from build123d import *

# Parameters (mm, degrees)
F0_R           = 8
F1_DEPTH       = 10
F2_SIZE        = 4
F3_SIZE        = 4
F4_D           = 3.3
F4_CSINK_D     = 6.72
F4_CSINK_ANGLE = 90
F6_D           = 5
F6_DEPTH       = 8
F6_TIP         = 1.5021515476


with BuildPart() as f1:
    # F0 (on Front) → F1 (new body)
    with BuildSketch(Plane.XZ):
        Polygon((-10, 0), (0, 0), (10, 0), (10, -10), (30, -10), (30, 0), (50, 0), (50, -10), (70, -10), (70, 0), (90, 0), (90, 15), (70, 15), (21, 258), (21, 300), (0, 300), (-21, 300), (-21, 258), (-70, 15), (-90, 15), (-90, 0), (-70, 0), (-70, -10), (-50, -10), (-50, 0), (-30, 0), (-30, -10), (-10, -10), align=None)
        with BuildLine():
            ThreePointArc((7.5, 50), (0, 42.5), (-7.5, 50))
            Line((-7.5, 50), (-7.5, 199.0483840028))
            ThreePointArc((-7.5, 199.0483840028), (0, 207.5601304887), (7.5, 199.0483840028))
            Line((7.5, 199.0483840028), (7.5, 50))
        make_face(mode=Mode.SUBTRACT)
        with Locations((0, 279)):
            Circle(F0_R, mode=Mode.SUBTRACT)
    extrude(amount=F1_DEPTH)

    # F2
    f2_edges = [f1.edges().sort_by_distance(p)[0] for p in [
        (21, -5, 300),
        (-21, -5, 300),
    ]]
    chamfer(f2_edges, length=F2_SIZE)

    # F3
    f3_edges = [f1.edges().sort_by_distance(p)[0] for p in [
        (-90, -5, 15),
        (90, -5, 15),
    ]]
    chamfer(f3_edges, length=F3_SIZE)

    # F4 (through all)
    with Locations(Plane(origin=(0, 0, 0), x_dir=(1, 0, 0), z_dir=(0, 1, 0))):
        with Locations((-15.5, -294.5), (15.5, -294.5), (15.5, -263.5), (-15.5, -263.5)):
            CounterSinkHole(F4_D / 2, F4_CSINK_D / 2, counter_sink_angle=F4_CSINK_ANGLE)

    # F6
    with Locations(Plane(origin=(0, 0, 0), x_dir=(1, 0, 0), z_dir=(0, 0, -1))):
        with Locations((-80, 5), (80, 5)):
            Hole(F6_D / 2, depth=F6_DEPTH)
            with Locations((0, 0, -(F6_DEPTH + F6_TIP / 2))):  # 118° drill point
                Cone(0, F6_D / 2, F6_TIP, mode=Mode.SUBTRACT)


solid = f1.part
Build history of the part. All positions in model axes, mm. A direction names the side the tool comes from. Round coordinates to 2 decimals unless told otherwise and drop trailing zeros. Write each loop counter-clockwise with the first axis right and the second up, starting at its lowest first coordinate (ties: lowest second). Pieces come first, ordered by that corner, then holes. Notation, with made-up numbers: (-26, 76.25) -> (-8, 76.25) arc R13 cw to (-8, 80.25) -> close; hole circle Ø2 at (8, -30). An arc over 180 degrees is marked (long way). Use one line per item in the form item = value.
Q1. Drill centre lines: L1, parallel to Z at x = 15.5, y = -6; L2, parallel to Y at x = 80, z = 6; L3, parallel to Z at x = -83, y = -9. Where is each one in solid material? Low to high.
Conclusion:
L1 = -10 to 261.85, 265.15 to 292.85, 296.15 to 300
L2 = -10 to -7.5, -2.5 to 0
L3 = 0 to 15
Q2. Band-saw the part on C-C, the plane x = -35. Write the cut outline in (y, z), then the cut area to 3 significant figures.
Conclusion:
outline = (-10, 0) -> (0, 0) -> (0, 188.57) -> (-10, 188.57) -> close
area = 1,890 mm²
Q3. Tool access for faces 1 (the flat face through (-78, -5, 15)), 2 (the cylindrical face through (0.16, -4.93, 42.5)), 3 (the flat face through (-30, -5, -5)): list every direction of +Z, -Z, +X, -X, +Y, -Y with a clear straight run to the whole face (end or side of a thin tool).
Conclusion:
face_1 = +Z, -X, +Y, -Y
face_2 = +Y, -Y
face_3 = -Z, +Y, -Y
Q4. Drop flat-ended pins along their axis: P1, Ø5, axis at y = -7, z = 272.5, coming from the +X side; P2, Ø4, axis at y = -6.5, z = 201, coming from the +X side; P3, Ø3, axis at x = -36.5, y = -7, coming from the -Z side; P4, Ø2, axis at x = 15.5, z = 294.5, coming from the -Y side. Give the stop position or say it passes through.
Conclusion:
P1 = 21
P2 = 32.9
P3 = 0
P4 = through
Q5. Band-saw the part on D-D, the plane z = 37. Write the cut outline in (x, y).
Conclusion:
outline = (-65.56, -10) -> (65.56, -10) -> (65.56, 0) -> (-65.56, 0) -> close
Q6. Two-plate mould, pull along X, no slides. Class faces 4 (the flat face through (-90, -5, 6)), 5 (the flat face through (40, -5, 0)), 6 (the flat face through (21, -5, 277)): released by +X, released by -X, zero draft, split by the parting line, or undercut.
Conclusion:
face_4 = released by -X
face_5 = undercut
face_6 = released by +X
Q7. Band-saw the part on A-A, the plane z = 279. Write the cut outline in (x, y), then the cut area to 3 significant figures.
Conclusion:
outline = (-21, -10) -> (-8, -10) -> (-8, 0) -> (-21, 0) -> close; (8, -10) -> (21, -10) -> (21, 0) -> (8, 0) -> close
area = 260 mm²
Q8. Band-saw the part on B-B, the plane z = 122. Write the cut outline in (x, y), then the cut area to 3 significant figures.
Conclusion:
outline = (-48.42, -10) -> (-7.5, -10) -> (-7.5, 0) -> (-48.42, 0) -> close; (7.5, -10) -> (48.42, -10) -> (48.42, 0) -> (7.5, 0) -> close
area = 818 mm²
